Verification items for the finished model (mm, model axes). Face numbers are marked on the shaded views. Give positions to 0.01 mm unless a question says otherwise; leave off trailing zeros. Order: outer loops, then holes, each group sorted by start corner. A loop starts at its lowest first (then second) coordinate and runs counter-clockwise, first axis right, second up. Notation, with made-up numbers: M 57.25,57.5 L 113.25,57.5 A20 cw 113.25,67.5 Z; hole C -31,75 d4. An arc over 180 degrees is marked long. Answer as a JSON object with one key per item and string values.
```python
from build123d import *

# Parameters (mm, degrees)
F0_R         = 19.5
F1_DEPTH     = 13
F2_R         = 18.5
F3_DEPTH     = 11
F4_W         = 45.72
F4_H         = 5.08
F5_DEPTH     = 3.81
F6_T1_DEPTH  = 52.07
F6_T3_DEPTH  = 11.43
F6_T8_ANGLE  = 183.7142551891
F6_T13_ANGLE = 183.7142551891
F7_R         = 0.7920917612
F8_DEPTH     = 3.81


# Not quite as in the source:
# - a fillet or chamfer that OpenCascade refuses, or shapes differently, is made with other operations: its cross-section is extruded or revolved along the edge and cut away or added


with BuildPart() as f1:
    # F0 (on Top) → F1 (new body)
    with BuildSketch(Plane.XY):
        Circle(F0_R)
    extrude(amount=F1_DEPTH)

    # F2 (on face) → F3 (cut)
    with BuildSketch(Plane.XY.offset(13)):
        Circle(F2_R)
    extrude(amount=-F3_DEPTH, mode=Mode.SUBTRACT)

    # F4 (on face) → F5 (join)
    with BuildSketch(Plane(origin=(0, 0, 0), x_dir=(1, 0, 0), z_dir=(0, 0, -1))):
        Rectangle(F4_W, F4_H)
    extrude(amount=F5_DEPTH)

    # F6: fillet of radius 1.27 on 6 edges, made by hand

    # F6_s2 → F6_t1 (cut)
    with BuildSketch(Plane.YZ.offset(-26.035)):
        with BuildLine():
            ThreePointArc((-2.54, -2.54), (-2.1680256121, -3.4380256121), (-1.27, -3.81))
            Line((-1.27, -3.81), (-2.54, -3.81))
            Line((-2.54, -3.81), (-2.54, -2.54))
        make_face()
        with BuildLine():
            ThreePointArc((2.54, -2.54), (2.1680256121, -3.4380256121), (1.27, -3.81))
            Line((1.27, -3.81), (2.54, -3.81))
            Line((2.54, -3.81), (2.54, -2.54))
        make_face()
    extrude(amount=F6_T1_DEPTH, mode=Mode.SUBTRACT)

    # F6_s4 → F6_t3 (cut)
    with BuildSketch(Plane.XZ.offset(-5.715)):
        with BuildLine():
            ThreePointArc((-21.59, 0), (-22.4880256121, -0.3719743879), (-22.86, -1.27))
            Line((-22.86, -1.27), (-22.86, 0))
            Line((-22.86, 0), (-21.59, 0))
        make_face()
        with BuildLine():
            ThreePointArc((21.59, 0), (22.4880256121, -0.3719743879), (22.86, -1.27))
            Line((22.86, -1.27), (22.86, 0))
            Line((22.86, 0), (21.59, 0))
        make_face()
    extrude(amount=F6_T3_DEPTH, mode=Mode.SUBTRACT)


with BuildPart() as f6_tool6:
    # F6_s7 → F6_t8 (revolve)
    with BuildSketch(Plane(origin=(0, 0, 0), x_dir=(0, 0, 1), z_dir=(-0.0324073159, -0.999474745, 0))):
        with BuildLine():
            ThreePointArc((1.27, -19.5), (0.3719743879, -19.1280256121), (0, -18.23))
            Line((0, -18.23), (0, -19.5))
            Line((0, -19.5), (1.27, -19.5))
        make_face()
    revolve(axis=Axis((0, 0, 0), (0, 0, 1)), revolution_arc=F6_T8_ANGLE)

    split(bisect_by=Plane.XZ.offset(-2.54), keep=Keep.BOTTOM)


with BuildPart() as f1_1:
    add(f1.part)

    # F6_t5: cut F6_tool6
    add(f6_tool6.part, mode=Mode.SUBTRACT)


with BuildPart() as f6_tool11:
    # F6_s12 → F6_t13 (revolve)
    with BuildSketch(Plane(origin=(0, 0, 0), x_dir=(0, 0, 1), z_dir=(0.0324073159, 0.999474745, 0))):
        with BuildLine():
            ThreePointArc((1.27, -19.5), (0.3719743879, -19.1280256121), (0, -18.23))
            Line((0, -18.23), (0, -19.5))
            Line((0, -19.5), (1.27, -19.5))
        make_face()
    revolve(axis=Axis((0, 0, 0), (0, 0, 1)), revolution_arc=F6_T13_ANGLE)

    split(bisect_by=Plane.XZ.offset(2.54), keep=Keep.TOP)


with BuildPart() as f1_2:
    add(f1_1.part)

    # F6_t10: cut F6_tool11
    add(f6_tool11.part, mode=Mode.SUBTRACT)

    # F7 (on face) → F8 (join, through all)
    with BuildSketch(Plane(origin=(0, 0, 0), x_dir=(1, 0, 0), z_dir=(0, 0, -1))):
        with Locations((10.5457008786, -6.0885632411)):
            Circle(F7_R)
        with Locations((-10.5457008786, -6.0885632411)):
            Circle(F7_R)
        with Locations((0, 12.1771264821)):
            Circle(F7_R)
    extrude(amount=F8_DEPTH)


solid = f1_2.part
```
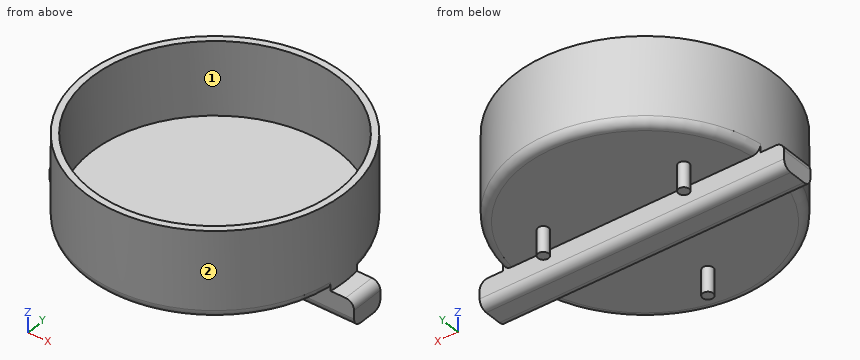
Q1. Gauge pin test, flat ends, axial feed: pin 1 Ø1 at (y, z) = (-0.5, 8) entering from +X; pin 2 Ø1.1 at (x, z) = (-1.5, -1) entering from -Y; pin 3 Ø12 at (x, y) = (-16.5, -9) entering from -Z. Record the tip position at first contact, or that the pin passes through.
Resolved:
{"pin 1": "stops at x = 19.5", "pin 2": "stops at y = -2.54", "pin 3": "stops at z = 0"}
Q2. Section check D-D on z = 5.75. Record the cut outline in (x, y).
Resolved:
{"outline": "C 0,0 d39; hole C 0,0 d37"}
Q3. Section check A-A on z = -0.5. Record the cut outline in (x, y), then the cut area to 3 significant figures.
Resolved:
{"outline": "M -22.6,-2.54 L 22.6,-2.54 L 22.6,2.54 L -22.6,2.54 Z; C -10.55,6.09 d1.58; C 0,-12.18 d1.58; C 10.55,6.09 d1.58", "area": "236 mm²"}
Q4. Section check C-C on y = 0. Record the cut outline in (x, z).
Resolved:
{"outline": "M -22.86,-3.81 L 22.86,-3.81 L 22.86,-1.27 A1.27 ccw 21.59,0 L 19.5,0 L 19.5,13 L 18.5,13 L 18.5,2 L -18.5,2 L -18.5,13 L -19.5,13 L -19.5,0 L -21.59,0 A1.27 ccw -22.86,-1.27 Z"}
Q5. Material ranges on L1, parallel to Y at x = 0, z = 5.25; L2, parallel to Z at x = 9.5, y = 6.5; L3, parallel to Y at x = -4, z = -2, recorded low to high.
Resolved:
{"L1": "y = -19.5 to -18.5, 18.5 to 19.5", "L2": "z = 0 to 2", "L3": "y = -2.54 to 2.54"}
Q6. Release check for a two-part mould opening along Y. For the marked faces 1 and 2 record: +Y half, -Y half, draft (parallel to the pull), parting line (faces both ways), or undercut.
Resolved:
{"face 1": "undercut", "face 2": "parting line"}
Q7. Section check B-B on x = 0. Record the cut outline in (y, z).
Resolved:
{"outline": "M -19.5,1.27 A1.27 ccw -18.23,0 L -12.97,0 L -12.97,-3.81 L -11.39,-3.81 L -11.39,0 L -2.54,0 L -2.54,-2.54 A1.27 ccw -1.27,-3.81 L 1.27,-3.81 A1.27 ccw 2.54,-2.54 L 2.54,0 L 18.23,0 A1.27 ccw 19.5,1.27 L 19.5,13 L 18.5,13 L 18.5,2 L -18.5,2 L -18.5,13 L -19.5,13 Z"}
